from build123d import *

# Parameters (mm, degrees)
F1_DEPTH    = 5.5
F2_R        = 27.25
F3_DEPTH    = 7
F4_R        = 22.5
F5_DEPTH    = 24
F6_R        = 20
F7_DEPTH    = 24
F8_R        = 16
F9_DEPTH    = 62.001
F10_R       = 18.5
F11_DEPTH   = 30
F12_SIZE    = 1
F13_SIZE2   = 2
F13_SIZE    = 5
F13_2_SIZE2 = 2
F13_2_SIZE  = 5


with BuildPart() as f1:
    # F0 (on Front) → F1 (new body, symmetric)
    with BuildSketch(Plane.XZ):
        Polygon((31.7542252363, 0.0501296029), (15.8336991085, 27.5250305336), (-15.9205261278, 27.4749009306), (-31.7542252363, -0.0501296029), (-15.8336991085, -27.5250305336), (15.9205261278, -27.4749009306), align=None)
    extrude(amount=F1_DEPTH, both=True)

    # F2 (on Front) → F3 (join, symmetric)
    with BuildSketch(Plane.XZ):
        Circle(F2_R)
    extrude(amount=F3_DEPTH, both=True)

    # F4 (on face) → F5 (join)
    with BuildSketch(Plane.XZ.offset(7)):
        Circle(F4_R)
    extrude(amount=F5_DEPTH)

    # F6 (on face) → F7 (join)
    with BuildSketch(Plane(origin=(0, 7, 0), x_dir=(-1, 0, 0), z_dir=(0, 1, 0))):
        Circle(F6_R)
    extrude(amount=F7_DEPTH)

    # F8 (on face) → F9 (cut, through all)
    with BuildSketch(Plane.XZ.offset(31)):
        Circle(F8_R)
    extrude(amount=-F9_DEPTH, mode=Mode.SUBTRACT)

    # F10 (on face) → F11 (cut)
    with BuildSketch(Plane.XZ.offset(31)):
        Circle(F10_R)
    extrude(amount=-F11_DEPTH, mode=Mode.SUBTRACT)

    # F12
    f12_edges = [f1.edges().sort_by_distance(p)[0] for p in [
        (-22.5, -31, 0),
        (20, 31, 0),
    ]]
    chamfer(f12_edges, length=F12_SIZE)

    # F13
    f13_edges = [f1.edges().sort_by_distance(p)[0] for p in [
        (-18.5, -31, 0),
    ]]
    f13_side = f1.faces().sort_by_distance((-18.5, -16, 0))[0]
    chamfer(f13_edges, length=F13_SIZE, length2=F13_SIZE2, reference=f13_side)

    # F13#2
    f13_2_edges = [f1.edges().sort_by_distance(p)[0] for p in [
        (-16, 31, 0),
    ]]
    f13_2_side = f1.faces().sort_by_distance((-16, 15, 0))[0]
    chamfer(f13_2_edges, length=F13_2_SIZE, length2=F13_2_SIZE2, reference=f13_2_side)


solid = f1.part
Work out the finished part from the listing and answer in its coordinate system (mm). A direction names the side the tool comes from. Round coordinates to 2 decimals unless told otherwise and drop trailing zeros. Loops run counter-clockwise (first coordinate to the right, second up) from the corner with the lowest first, then second, coordinate; pieces in that order, holes last. Notation, with made-up numbers: (56.25, 14.5) - (60.25, 14.5) arc R9 ccw to (60.25, 25.5) - close; hole circle Ø8 at (14.25, 3.25). An arc over 180 degrees is marked (long way). One line per item, written item: value.
Q1. Each of these flat-tipped pins is pushed along its axis until it touches: pin 1 Ø12 at (x, y) = (-5, -15) entering from +Z; pin 2 Ø6 at (x, y) = (0.5, 12) entering from +Z; pin 3 Ø12 at (x, y) = (22.5, -8) entering from -Z; pin 4 Ø1.5 at (x, y) = (-22.5, 24) entering from -Z. Where does it stop, or does it pass through?
Check values:
pin 1: z = 22.5
pin 2: z = 20
pin 3: z = -25.52
pin 4: through
Q2. Find section B-B on z = 24. Give the vertices of the cut face in (x, y).
Check values:
outline: (-17.92, -5.5) - (-12.91, -5.5) - (-12.91, -7) - (12.91, -7) - (12.91, -5.5) - (17.88, -5.5) - (17.88, 5.5) - (12.91, 5.5) - (12.91, 7) - (-12.91, 7) - (-12.91, 5.5) - (-17.92, 5.5) - close
Q3. The mould has two halves that part along Z. Classify faces 1 (the flat face through (28, -5.5, 0)), 2 (the flat face through (-23.905, -0.077, -13.595)), 3 (the conical face through (-4.04, -26.31, -18.18)): +Z half, -Z half, draft (parallel to the pull), parting line (faces both ways), or undercut.
Check values:
face 1: draft
face 2: -Z half
face 3: undercut
Q4. Find section C-C on x = 25.5. Give the vertices of the cut face in (y, z), and give its area (3 significant figures).
Check values:
outline: (-7, -9.61) - (-5.5, -9.61) - (-5.5, -10.82) - (5.5, -10.82) - (5.5, -9.61) - (7, -9.61) - (7, 9.61) - (5.5, 9.61) - (5.5, 10.84) - (-5.5, 10.84) - (-5.5, 9.61) - (-7, 9.61) - close
area: 296 mm2
Q5. Straight lines are drawn through the part: probe 1 along Z at (x, y) = (0, 12); probe 2 along Y at (x, z) = (12, -24); probe 3 along Z at (x, y) = (0, -20). For each, find the intervals that lie inside material, in ascending order.
Check values:
probe 1: -20 to -16, 16 to 20
probe 2: -7 to 7
probe 3: -22.5 to -18.5, 18.5 to 22.5
Q6. For faces 4 (the flat face through (-14.3, 7, 14.3)), 5 (the cylindrical face through (-3.47, 12.31, -15.62)), 6 (the cylindrical face through (-21.625, -6.26, -16.581)), determine the directions among +Z, -Z, +X, -X, +Y, -Y from which every point of the face is accessible in a straight line to the end or side of a thin tool.
Check values:
face 4: +Y
face 5: +Y, -Y
face 6: -Y
Q7. Find section A-A on y = -19. Give the vertices of the cut face in (x, z), and give its area (3 significant figures).
Check values:
outline: circle Ø45 at (0, 0); hole circle Ø37 at (0, 0)
area: 515 mm2
